Build history of the part. All positions in model axes, mm. Face numbers are marked on the shaded views. Give positions to 0.01 mm unless a question says otherwise; leave off trailing zeros. Loops run counter-clockwise (first coordinate to the right, second up) from the corner with the lowest first, then second, coordinate; pieces in that order, holes last. Notation, with made-up numbers: (83, 50.25) - (124, 50.25) arc R14 cw to (124, 58.25) - close; hole circle Ø8 at (78, 79). An arc over 180 degrees is marked (long way). Return JSON: item names as keys, results as strings. Group by question number.
1) Mould opens along X. For the marked faces 1, 2 and 3 say: released by +X, released by -X, zero draft, split by the parting line, or undercut.
2) Slice it at A-A (x = 0). List the corners of the cut face in (y, z), and give its area (3 significant figures).
3) Slice it at B-B (z = -180.5). List the corners of the cut face in (x, y), and give its area (3 significant figures).
4) Slice it at D-D (x = -15.5). List the corners of the cut face in (y, z), and give its area (3 significant figures).
5) Slice it at C-C (y = 1.25). Count the separate pieces of the cut face and the enclosed holes in it, and give its area (3 significant figures).
6) Drop flat-ended pins along their axis: pin 1 (3 mm diameter, centred on y = -13, z = -194.5, fed in from -X); pin 2 (12 mm diameter, centred on x = 30.5, z = -183.5, fed in from -Y); pin 3 (5 mm diameter, centred on x = 10, y = 1, fed in from +Z); pin 4 (5.5 mm diameter, centred on x = -40, y = -7.5, fed in from -Z). Give the stop position or say it passes through.
7) Drill centre lines: probe 1 along Y at (x, z) = (0, -201); probe 2 along Y at (x, z) = (17, -188.75); probe 3 along Z at (x, y) = (16, -2.75). Where is each one in solid material? Low to high. Write a range as from..to.
Autodesk Inventor part; units mm, degrees
ref_plane "YZ Plane" through (0, 0, 0) normal (1, 0, 0) x (0, 1, 0)
ref_plane "XZ Plane" through (0, 0, 0) normal (0, 1, 0) x (-1, 0, 0)
sketch "Sketch1" plane through (0, 0, 0) normal (0, 1, 0) x (-1, 0, 0)
  circle A0 centre (0, 0) radius 200
  line L0 (0, 0) -> (0, -200)
  line L1 (0, 0) -> (-61.8034, -190.2113)
  line L2 (0, 0) -> (200, 0) construction
  line L3 (-61.8034, -190.2113) -> (0, 0)
  line L4 (0, 0) -> (61.8034, -190.2113)
  line L5 (0, 0) -> (200, 0) construction
  arc A1 (-61.8034, -190.2113) -> (61.8034, -190.2113) centre (0, 0) ccw
  line L6 (-61.8034, -190.2113) -> (-62.7304, -193.0645)
  line L7 (61.8034, -190.2113) -> (62.7304, -193.0645)
  line L8 (0, -200) -> (0, -203)
  arc A2 (-62.7304, -193.0645) -> (62.7304, -193.0645) centre (0, 0) ccw
  dimension "d0" = 400
  dimension "d1" = 108
  dimension "d2" = 72
  dimension "d4" = 3
  dimension "d5" = 3
  dimension "d6" = 3
extrude "Extrusion1" add sketch "Sketch1" along normal blind 3 and the other way blind 15 contours A0 L8 A2 L6 | L7 A2 L8 A0
sketch "Sketch3" plane through (0, 3, 0) normal (0, 1, 0) x (1, 0, 0)
  arc A0 (62.7304, 193.0645) -> (-62.7304, 193.0645) centre (0, 0) ccw
  line L0 (-62.7304, 193.0645) -> (-57.1681, 175.9455)
  line L1 (-62.7304, 193.0645) -> (-61.8034, 190.2113)
  line L2 (0, 203) -> (0, 185)
  line L3 (61.8034, 190.2113) -> (62.7304, 193.0645)
  line L4 (62.7304, 193.0645) -> (57.1681, 175.9455)
  arc A1 (57.1681, 175.9455) -> (-57.1681, 175.9455) centre (0, 0) ccw
  point P0 (0, 0)
  dimension "d12" = 18
  dimension "d13" = 18
  dimension "d14" = 18
extrude "Extrusion2" add sketch "Sketch3" against normal blind 3
sketch "Sketch4" plane through (0, 3, 0) normal (0, 1, 0) x (1, 0, 0)
  arc A0 (62.7304, 193.0645) -> (-62.7304, 193.0645) centre (0, 0) ccw
  line L0 (0, 203) -> (0, 200)
  line L1 (0, 200) -> (0, 192.5)
  circle A1 centre (0, 192.5) radius 1.75
  line L2 (57.1681, 175.9455) -> (62.7304, 193.0645)
  line L3 (62.7304, 193.0645) -> (57.1681, 175.9455)
  line L4 (-62.7304, 193.0645) -> (-57.1681, 175.9455)
  line L5 (-62.7304, 193.0645) -> (-57.1681, 175.9455)
  line L6 (-57.1681, 175.9455) -> (-62.7304, 193.0645)
  line L7 (-62.7304, 193.0645) -> (-61.8034, 190.2113)
  line L8 (-61.8034, 190.2113) -> (-59.4858, 183.0784)
  line L9 (62.7304, 193.0645) -> (61.8034, 190.2113)
  line L10 (61.8034, 190.2113) -> (59.4858, 183.0784)
  arc A2 (59.4858, 183.0784) -> (-59.4858, 183.0784) centre (0, 0) ccw
  line L11 (0, 192.5) -> (39.7835, 188.3442)
  line L12 (39.7835, 188.3442) -> (0, 192.5)
  line L13 (0, 192.5) -> (-39.7835, 188.3442)
  circle A3 centre (39.7835, 188.3442) radius 1.75
  circle A4 centre (-39.7835, 188.3442) radius 1.75
  point P0 (0, 0)
  dimension "d17" = 3
  dimension "d18" = 7.5
  dimension "d19" = 3.5
  dimension "d28" = 3
  dimension "d29" = 7.5
  dimension "d30" = 3
  dimension "d31" = 7.5
  dimension "d32" = 40
  dimension "d33" = 40
  dimension "d34" = 3.5
  dimension "d35" = 3.5
extrude "Extrusion3" cut sketch "Sketch4" against normal blind 3 contours A1 A2 L1 | L1 A2 A1 | A3 L11 A2 | A2 A3 | L13 A1 A2 | A2 A1 L11 | L11 A1 L13 | L11 A3 A2 | A4 A2 | A2 L13 A4 | A4 L13 A2
ref_plane "Work Plane1" through (0, 0, -200) normal (0, 0, 1) x (1, 0, 0)
sketch "Sketch6" plane through (0, 0, -200) normal (0, 0, 1) x (1, 0, 0)
  line L0 (62.7304, 3) -> (-62.7304, 3)
  line L1 (0, 3) -> (0, -15)
  line L2 (-62.7304, -15) -> (62.7304, -15)
  line L3 (0, 3) -> (0, -15)
  line L4 (61.8034, -15) -> (-61.8034, -15)
  line L5 (0, 3) -> (0, 0)
  line L6 (0, 0) -> (0, -7.5)
  circle A0 centre (0, -7.5) radius 1.75
  line L7 (0, -7.5) -> (-40, -7.5)
  line L8 (-40, -7.5) -> (40, -7.5)
  circle A1 centre (-40, -7.5) radius 1.75
  circle A2 centre (40, -7.5) radius 1.75
  dimension "d23" = 3
  dimension "d24" = 7.5
  dimension "d25" = 3.5
  dimension "d36" = 40
  dimension "d37" = 80
  dimension "d38" = 3.5
  dimension "d39" = 3.5
extrude "Extrusion4" cut sketch "Sketch6" against normal mid plane 10
properties part number "Casing_holder_bottom"
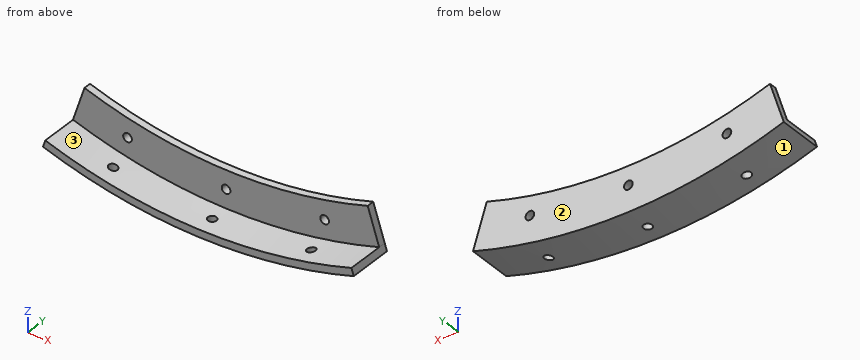
Results:
{
 "1": {"face 1": "split by the parting line", "face 2": "zero draft", "face 3": "undercut"},
 "2": {"outline": "(-15, -203) - (-9.25, -203) - (-9.25, -200) - (-15, -200) - close; (-5.75, -203) - (3, -203) - (3, -194.25) - (0, -194.25) - (0, -200) - (-5.75, -200) - close; (0, -190.75) - (3, -190.75) - (3, -185) - (0, -185) - close", "area": "78.0 mm2"},
 "3": {"outline": "(-58.65, 0) - (-40.56, 0) - (-40.56, 3) - (-58.65, 3) - close; (40.56, 0) - (58.65, 0) - (58.65, 3) - (40.56, 3) - close", "area": "109 mm2"},
 "4": {"outline": "(-15, -202.41) - (3, -202.41) - (3, -184.35) - (0, -184.35) - (0, -199.4) - (-15, -199.4) - close", "area": "99.3 mm2"},
 "5": {"separate pieces": "1", "enclosed holes": "3", "area": "2,170 mm2"},
 "6": {"pin 1": "x = -62.73", "pin 2": "y = 0", "pin 3": "z = -184.58", "pin 4": "z = -199.55"},
 "7": {"probe 1": "-15..-9.25, -5.75..3", "probe 2": "0..3", "probe 3": "-202.37..-199.36"}
}
